from build123d import *

# Parameters (mm, degrees)
SKETCH_1_W          = 9
SKETCH_1_H          = 6.5
EXTRUDE_1_DEPTH     = 430
SKETCH_2_R          = 1.750000006
CUT_EXTRUDE_1_DEPTH = 341.826868595
SKETCH_3_R          = 3.000000006
CUT_EXTRUDE_2_DEPTH = 3.5


with BuildPart() as part:
    # 草图1 → 凸台-拉伸1 (new body)
    with BuildSketch(Plane.XY.offset(-89.264832522)):
        Rectangle(SKETCH_1_W, SKETCH_1_H)
    extrude(amount=EXTRUDE_1_DEPTH)

    # 草图2 → 切除-拉伸1 (cut, through all)
    with BuildSketch(Plane(origin=(0, 3.25, 0), x_dir=(1, 0, 0), z_dir=(0, 1, 0))):
        with Locations(Location((0, 81.764832522, 0), (0, 0, 270))):
            Circle(SKETCH_2_R)
        with Locations(Location((0, 61.764832522, 0), (0, 0, 270))):
            Circle(SKETCH_2_R)
        with Locations(Location((0, 41.764832522, 0), (0, 0, 270))):
            Circle(SKETCH_2_R)
        with Locations(Location((0, 21.764832522, 0), (0, 0, 270))):
            Circle(SKETCH_2_R)
        with Locations(Location((0, 1.764832522, 0), (0, 0, 270))):
            Circle(SKETCH_2_R)
        with Locations(Location((0, -18.235167478, 0), (0, 0, 270))):
            Circle(SKETCH_2_R)
        with Locations(Location((0, -38.235167478, 0), (0, 0, 270))):
            Circle(SKETCH_2_R)
        with Locations(Location((0, -58.235167478, 0), (0, 0, 270))):
            Circle(SKETCH_2_R)
        with Locations(Location((0, -78.235167478, 0), (0, 0, 270))):
            Circle(SKETCH_2_R)
        with Locations(Location((0, -98.235167478, 0), (0, 0, 270))):
            Circle(SKETCH_2_R)
        with Locations(Location((0, -118.235167478, 0), (0, 0, 270))):
            Circle(SKETCH_2_R)
        with Locations(Location((0, -138.235167478, 0), (0, 0, 270))):
            Circle(SKETCH_2_R)
        with Locations(Location((0, -158.235167478, 0), (0, 0, 270))):
            Circle(SKETCH_2_R)
        with Locations(Location((0, -178.235167478, 0), (0, 0, 270))):
            Circle(SKETCH_2_R)
        with Locations(Location((0, -198.235167478, 0), (0, 0, 270))):
            Circle(SKETCH_2_R)
        with Locations(Location((0, -218.235167478, 0), (0, 0, 270))):
            Circle(SKETCH_2_R)
        with Locations(Location((0, -238.235167478, 0), (0, 0, 270))):
            Circle(SKETCH_2_R)
        with Locations(Location((0, -258.235167478, 0), (0, 0, 270))):
            Circle(SKETCH_2_R)
        with Locations(Location((0, -278.235167478, 0), (0, 0, 270))):
            Circle(SKETCH_2_R)
        with Locations(Location((0, -298.235167478, 0), (0, 0, 270))):
            Circle(SKETCH_2_R)
        with Locations(Location((0, -318.235167478, 0), (0, 0, 270))):
            Circle(SKETCH_2_R)
        with Locations(Location((0, -338.235167478, 0), (0, 0, 270))):
            Circle(SKETCH_2_R)
        with Locations((0, -358.235167478)):
            Circle(SKETCH_2_R)
        with Locations((0, -378.235167478)):
            Circle(SKETCH_2_R)
        with Locations((0, -398.235167478)):
            Circle(SKETCH_2_R)
        with Locations((0, -418.235167478)):
            Circle(SKETCH_2_R)
        with Locations((0, -438.235167478)):
            Circle(SKETCH_2_R)
        with Locations((0, -458.235167478)):
            Circle(SKETCH_2_R)
        with Locations((0, -478.235167478)):
            Circle(SKETCH_2_R)
        with Locations((0, -498.235167478)):
            Circle(SKETCH_2_R)
        with Locations((0, -518.235167478)):
            Circle(SKETCH_2_R)
        with Locations((0, -538.235167478)):
            Circle(SKETCH_2_R)
        with Locations((0, -558.235167478)):
            Circle(SKETCH_2_R)
        with Locations((0, -578.235167478)):
            Circle(SKETCH_2_R)
        with Locations((0, -598.235167478)):
            Circle(SKETCH_2_R)
        with Locations((0, -618.235167478)):
            Circle(SKETCH_2_R)
        with Locations((0, -638.235167478)):
            Circle(SKETCH_2_R)
        with Locations((0, -658.235167478)):
            Circle(SKETCH_2_R)
        with Locations((0, -678.235167478)):
            Circle(SKETCH_2_R)
        with Locations((0, -698.235167478)):
            Circle(SKETCH_2_R)
        with Locations((0, -718.235167478)):
            Circle(SKETCH_2_R)
        with Locations((0, -738.235167478)):
            Circle(SKETCH_2_R)
        with Locations((0, -758.235167478)):
            Circle(SKETCH_2_R)
        with Locations((0, -778.235167478)):
            Circle(SKETCH_2_R)
        with Locations((0, -798.235167478)):
            Circle(SKETCH_2_R)
        with Locations((0, -818.235167478)):
            Circle(SKETCH_2_R)
        with Locations((0, -838.235167478)):
            Circle(SKETCH_2_R)
        with Locations((0, -858.235167478)):
            Circle(SKETCH_2_R)
        with Locations((0, -878.235167478)):
            Circle(SKETCH_2_R)
        with Locations((0, -898.235167478)):
            Circle(SKETCH_2_R)
        with Locations((0, -918.235167478)):
            Circle(SKETCH_2_R)
        with Locations((0, -938.235167478)):
            Circle(SKETCH_2_R)
        with Locations((0, -958.235167478)):
            Circle(SKETCH_2_R)
        with Locations((0, -978.235167478)):
            Circle(SKETCH_2_R)
        with Locations((0, -998.235167478)):
            Circle(SKETCH_2_R)
        with Locations((0, -1018.235167478)):
            Circle(SKETCH_2_R)
        with Locations((0, -1038.235167478)):
            Circle(SKETCH_2_R)
        with Locations((0, -1058.235167478)):
            Circle(SKETCH_2_R)
        with Locations((0, -1078.235167478)):
            Circle(SKETCH_2_R)
        with Locations((0, -1098.235167478)):
            Circle(SKETCH_2_R)
    extrude(amount=-CUT_EXTRUDE_1_DEPTH, mode=Mode.SUBTRACT)

    # 草图3 → 切除-拉伸2 (cut)
    with BuildSketch(Plane(origin=(0, 3.25, 0), x_dir=(1, 0, 0), z_dir=(0, 1, 0))):
        with Locations(Location((0, 81.764832522, 0), (0, 0, 270))):
            Circle(SKETCH_3_R)
        with Locations(Location((0, 61.764832522, 0), (0, 0, 270))):
            Circle(SKETCH_3_R)
        with Locations(Location((0, 41.764832522, 0), (0, 0, 270))):
            Circle(SKETCH_3_R)
        with Locations(Location((0, 21.764832522, 0), (0, 0, 270))):
            Circle(SKETCH_3_R)
        with Locations(Location((0, 1.764832522, 0), (0, 0, 270))):
            Circle(SKETCH_3_R)
        with Locations(Location((0, -18.235167478, 0), (0, 0, 270))):
            Circle(SKETCH_3_R)
        with Locations(Location((0, -38.235167478, 0), (0, 0, 270))):
            Circle(SKETCH_3_R)
        with Locations(Location((0, -58.235167478, 0), (0, 0, 270))):
            Circle(SKETCH_3_R)
        with Locations(Location((0, -78.235167478, 0), (0, 0, 270))):
            Circle(SKETCH_3_R)
        with Locations(Location((0, -98.235167478, 0), (0, 0, 270))):
            Circle(SKETCH_3_R)
        with Locations(Location((0, -118.235167478, 0), (0, 0, 270))):
            Circle(SKETCH_3_R)
        with Locations(Location((0, -138.235167478, 0), (0, 0, 270))):
            Circle(SKETCH_3_R)
        with Locations(Location((0, -158.235167478, 0), (0, 0, 270))):
            Circle(SKETCH_3_R)
        with Locations(Location((0, -178.235167478, 0), (0, 0, 270))):
            Circle(SKETCH_3_R)
        with Locations(Location((0, -198.235167478, 0), (0, 0, 270))):
            Circle(SKETCH_3_R)
        with Locations(Location((0, -218.235167478, 0), (0, 0, 270))):
            Circle(SKETCH_3_R)
        with Locations(Location((0, -238.235167478, 0), (0, 0, 270))):
            Circle(SKETCH_3_R)
        with Locations(Location((0, -258.235167478, 0), (0, 0, 270))):
            Circle(SKETCH_3_R)
        with Locations(Location((0, -278.235167478, 0), (0, 0, 270))):
            Circle(SKETCH_3_R)
        with Locations(Location((0, -298.235167478, 0), (0, 0, 270))):
            Circle(SKETCH_3_R)
        with Locations(Location((0, -318.235167478, 0), (0, 0, 270))):
            Circle(SKETCH_3_R)
        with Locations((0, -338.235167478)):
            Circle(SKETCH_3_R)
        with Locations((0, -358.235167478)):
            Circle(SKETCH_3_R)
        with Locations((0, -378.235167478)):
            Circle(SKETCH_3_R)
        with Locations((0, -398.235167478)):
            Circle(SKETCH_3_R)
        with Locations((0, -418.235167478)):
            Circle(SKETCH_3_R)
        with Locations((0, -438.235167478)):
            Circle(SKETCH_3_R)
        with Locations((0, -458.235167478)):
            Circle(SKETCH_3_R)
        with Locations((0, -478.235167478)):
            Circle(SKETCH_3_R)
        with Locations((0, -498.235167478)):
            Circle(SKETCH_3_R)
        with Locations((0, -518.235167478)):
            Circle(SKETCH_3_R)
        with Locations((0, -538.235167478)):
            Circle(SKETCH_3_R)
        with Locations((0, -558.235167478)):
            Circle(SKETCH_3_R)
        with Locations((0, -578.235167478)):
            Circle(SKETCH_3_R)
        with Locations((0, -598.235167478)):
            Circle(SKETCH_3_R)
        with Locations((0, -618.235167478)):
            Circle(SKETCH_3_R)
        with Locations((0, -638.235167478)):
            Circle(SKETCH_3_R)
        with Locations((0, -658.235167478)):
            Circle(SKETCH_3_R)
        with Locations((0, -678.235167478)):
            Circle(SKETCH_3_R)
        with Locations((0, -698.235167478)):
            Circle(SKETCH_3_R)
        with Locations((0, -718.235167478)):
            Circle(SKETCH_3_R)
        with Locations((0, -738.235167478)):
            Circle(SKETCH_3_R)
        with Locations((0, -758.235167478)):
            Circle(SKETCH_3_R)
        with Locations((0, -778.235167478)):
            Circle(SKETCH_3_R)
        with Locations((0, -798.235167478)):
            Circle(SKETCH_3_R)
        with Locations((0, -818.235167478)):
            Circle(SKETCH_3_R)
        with Locations((0, -838.235167478)):
            Circle(SKETCH_3_R)
        with Locations((0, -858.235167478)):
            Circle(SKETCH_3_R)
        with Locations((0, -878.235167478)):
            Circle(SKETCH_3_R)
        with Locations((0, -898.235167478)):
            Circle(SKETCH_3_R)
        with Locations((0, -918.235167478)):
            Circle(SKETCH_3_R)
        with Locations((0, -938.235167478)):
            Circle(SKETCH_3_R)
        with Locations((0, -958.235167478)):
            Circle(SKETCH_3_R)
        with Locations((0, -978.235167478)):
            Circle(SKETCH_3_R)
        with Locations((0, -998.235167478)):
            Circle(SKETCH_3_R)
        with Locations((0, -1018.235167478)):
            Circle(SKETCH_3_R)
        with Locations((0, -1038.235167478)):
            Circle(SKETCH_3_R)
        with Locations((0, -1058.235167478)):
            Circle(SKETCH_3_R)
        with Locations((0, -1078.235167478)):
            Circle(SKETCH_3_R)
        with Locations((0, -1098.235167478)):
            Circle(SKETCH_3_R)
    extrude(amount=-CUT_EXTRUDE_2_DEPTH, mode=Mode.SUBTRACT)


solid = part.part
Source: CAD feature listing. Evaluate the final solid. Frame: model axes, mm. Give positions to 0.01 mm unless a question says otherwise; leave off trailing zeros. Return JSON: item names as keys, results as strings. Group by question number.
1. Section A-A, the plane y = -2. Count the separate pieces of the cut face and the enclosed holes in it, then the cut area to 3 significant figures.
2. Material intervals for line 1 (Y direction, x = -0.5, z = 96); line 2 (X direction, y = 2.75, z = 20); line 3 (X direction, y = -1, z = 79), sorted ascending. Write a range as from..to.
3. Pin query (flat end, axial travel): pin 1 Ø1.8 at (x, z) = (1, 198.5) entering from +Y. Return the tip coordinate at first contact, or that it passes through.
Determined:
{
 "1": {"separate pieces": "1", "enclosed holes": "22", "area": "3,660 mm2"},
 "2": {"line 1": "y = -3.25..-0.25", "line 2": "x = -4.5..-2.43, 2.43..4.5", "line 3": "x = -4.5..-1.57, 1.57..4.5"},
 "3": {"pin 1": "stops at y = -0.25"}
}
